Check sheet for the drawn part. Datum: minimum x, y, z corner. Units: mm. Give positions to 0.01 mm unless a question says otherwise; leave off trailing zeros. Order: outer loops, then holes, each group sorted by start corner. A loop starts at its lowest first (then second) coordinate and runs counter-clockwise, first axis right, second up. Notation, with made-up numbers: (9.5, -14.5) -> (21.5, -14.5) arc R18 cw to (21.5, 20.5) -> close; hole circle Ø9 at (-30, 63). An arc over 180 degrees is marked (long way). Return JSON: item names as keys, results as strings. Group by question number.
(1) Depth check by flat-ended pin: pin 1 Ø12.5 at (x, y) = (138, 618.5) entering from -Z; pin 2 Ø12.5 at (x, z) = (137, 564) entering from -Y; pin 3 Ø10 at (y, z) = (666, 299.5) entering from +X. Enter the tip coordinate at first touch or a pass-through.
(2) Cross-section at C-C on z = 189. Enter the section's corners in (x, y), then the cut area to 3 significant figures.
(3) Cross-section at D-D on y = 348.5. Enter the section's corners in (x, z), then the cut area to 3 significant figures.
(4) Cross-section at A-A on x = 141. Enter the section's corners in (y, z), then the cut area to 3 significant figures.
(5) Release check for a two-part mould opening along Z. For the marked faces 1, 2, 3 and 4 record: pulls with the +Z half, pulls with the -Z half, needs draft (parallel to the pull), parting line crosses it, or undercut.
(6) Cross-section at B-B on y = 450. Enter the section's corners in (x, z).
(7) Thickness scan on line 1 along Z through (x, y) = (142.5, 39); line 2 along X through (y, z) = (420, 343); line 3 along Z through (x, y) = (129, 355.5). Record the ranges inside material, lowest first.
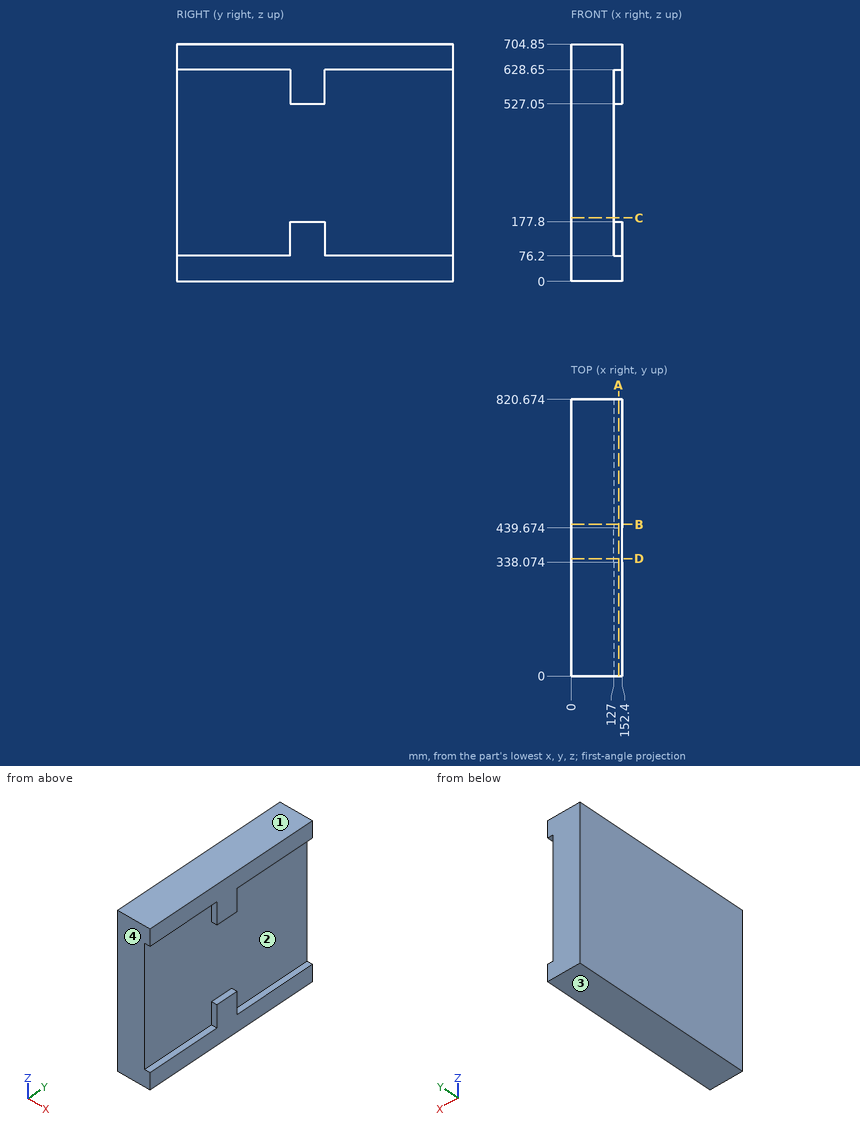
Verdict:
{
 "1": {"pin 1": "z = 0", "pin 2": "y = 338.07", "pin 3": "x = 127"},
 "2": {"outline": "(0, 0) -> (127, 0) -> (127, 820.67) -> (0, 820.67) -> close", "area": "104,000 mm²"},
 "3": {"outline": "(0, 0) -> (152.4, 0) -> (152.4, 177.8) -> (127, 177.8) -> (127, 527.05) -> (152.4, 527.05) -> (152.4, 704.85) -> (0, 704.85) -> close", "area": "98,500 mm²"},
 "4": {"outline": "(0, 0) -> (820.67, 0) -> (820.67, 76.2) -> (439.67, 76.2) -> (439.67, 177.8) -> (338.07, 177.8) -> (338.07, 76.2) -> (0, 76.2) -> close; (0, 628.65) -> (338.07, 628.65) -> (338.07, 527.05) -> (439.67, 527.05) -> (439.67, 628.65) -> (820.67, 628.65) -> (820.67, 704.85) -> (0, 704.85) -> close", "area": "146,000 mm²"},
 "5": {"face 1": "pulls with the +Z half", "face 2": "undercut", "face 3": "pulls with the -Z half", "face 4": "needs draft"},
 "6": {"outline": "(0, 0) -> (152.4, 0) -> (152.4, 76.2) -> (127, 76.2) -> (127, 628.65) -> (152.4, 628.65) -> (152.4, 704.85) -> (0, 704.85) -> close"},
 "7": {"line 1": "0 to 76.2, 628.65 to 704.85", "line 2": "0 to 127", "line 3": "0 to 177.8, 527.05 to 704.85"}
}
